Source: CAD feature listing. Evaluate the final solid. Frame: model axes, mm. Round coordinates to 2 decimals unless told otherwise and drop trailing zeros. Write each loop counter-clockwise with the first axis right and the second up, starting at its lowest first coordinate (ties: lowest second). Pieces come first, ordered by that corner, then holes. Notation, with made-up numbers: (-32, 35) -> (-26, 35) arc R25 ccw to (-26, 61) -> close; hole circle Ø10 at (60.25, 22). An arc over 180 degrees is marked (long way). Return JSON: item names as keys, results as strings. Group by question number.
Autodesk Inventor part; units mm, degrees
ref_plane "Work Plane1" through (-3.5125, -3.5125, 37.5) normal (0, 0, 1) x (0.9087, 0.4175, 0)
ref_plane "Work Plane2" through (-0.9, -20.4499, 62.8) normal (0, 0, 1) x (1, 0, 0)
ref_plane "YZ Plane" through (0, 0, 0) normal (1, 0, 0) x (0, 1, 0)
sketch "Sketch1" plane through (0, 0, 0) normal (0, 0, 1) x (1, 0, 0)
  circle A0 centre (0, 0) radius 6
  circle A1 centre (0, 0) radius 2
  point P0 (0, 0)
  dimension "d0" = 4
ref_plane "Work Plane1" through (-3.5125, -3.5125, 37.5) normal (0, 0, 1) x (0.9087, 0.4175, 0)
extrude "Extrusion1" add sketch "Sketch1" along normal up to surface (37.5 mm away) contours A1
sketch "Sketch2" plane through (0, 0, 37.5) normal (0, 0, 1) x (1, 0, 0)
  circle A0 centre (0, 0) radius 2
  point P0 (0, 0)
extrude "Extrusion2" add sketch "Sketch2" along normal blind 2 draft -40
sketch "Sketch3" plane through (0, 0, 39.5) normal (0, 0, 1) x (1, 0, 0)
  circle A0 centre (0, 0) radius 0.3218
  point P0 (0, 0)
ref_plane "Work Plane2" through (-0.9, -20.4499, 62.8) normal (0, 0, 1) x (1, 0, 0)
extrude "Extrusion3" add sketch "Sketch3" along normal up to surface (23.3 mm away)
properties part number "cellSTORM_laserbeam"
Item 1: Material intervals for probe 1 along Y at (x, z) = (0.05, 51.5); probe 2 along X at (y, z) = (0.15, 7); probe 3 along Z at (x, y) = (0.4, 0.4), sorted ascending.
Item 2: First-contact query: pin 1 Ø1 at (x, z) = (-1.5, 53.5) entering from +Y; pin 2 Ø1.5 at (x, y) = (0, 1.5) entering from +Z. Flat tips, straight axial feed; report the tip coordinate or a pass-through.
Item 3: Cut plane B-B on z = 53. Output: boundary loops of the cut face in (x, y), and give its area (3 significant figures).
Item 4: Cut plane A-A on z = 33. Output: boundary loops of the cut face in (x, y).
Here are the results:
{
 "1": {"probe 1": "y = -0.32 to 0.32", "probe 2": "x = -1.99 to 1.99", "probe 3": "z = 0 to 39.21"},
 "2": {"pin 1": "passes through", "pin 2": "stops at z = 38.99"},
 "3": {"outline": "circle Ø0.64 at (0, 0)", "area": "0.325 mm^2"},
 "4": {"outline": "circle Ø4 at (0, 0)"}
}
